from build123d import *

# Parameters (mm, degrees)
F0_W      = 660.4
F0_H      = 304.8
F1_DEPTH  = 6.35
F2_W      = 50.8
F2_H      = 50.8
F3_DEPTH  = 6.35
F4_W      = 50.8
F4_H      = 6.35
F5_W      = 50.8
F5_H      = 6.35
F6_W      = 50.8
F6_H      = 6.35
F7_DEPTH  = 44.45
F8_W      = 101.6
F8_H      = 50.8
F9_DEPTH  = 9.525
F10_W     = 101.6
F10_H     = 50.8
F11_DEPTH = 25.4
F12_W     = 9.525
F12_H     = 50.8
F13_DEPTH = 76.2
F14_W     = 9.525
F14_H     = 50.8
F15_DEPTH = 117.475
F16_R     = 6.35
F17_DEPTH = 25.4
F18_W     = 76.2
F18_H     = 9.525
F19_DEPTH = 76.2
F21_DEPTH = 25.4


with BuildPart() as f1:
    # F0 (on Front) → F1 (new body)
    with BuildSketch(Plane.XZ):
        Rectangle(F0_W, F0_H)
    extrude(amount=F1_DEPTH)

    # F2 (on face) → F3 (join)
    with BuildSketch(Plane.XZ.offset(6.35)):
        with Locations((165.1, -127)):
            Rectangle(F2_W, F2_H)
        with Locations((0, -127)):
            Rectangle(F2_W, F2_H)
        with Locations((-177.8, -127)):
            Rectangle(F2_W, F2_H)
    extrude(amount=F3_DEPTH)

    # F4 (on face) + F5 (on face) + F6 (on face) → F7 (join)
    with BuildSketch(Plane.XZ.offset(12.7)):
        with Locations((-177.8, -149.225)):
            Rectangle(F4_W, F4_H)
    with BuildSketch(Plane.XZ.offset(12.7)):
        with Locations((0, -149.225)):
            Rectangle(F5_W, F5_H)
    with BuildSketch(Plane.XZ.offset(12.7)):
        with Locations((165.1, -149.225)):
            Rectangle(F6_W, F6_H)
    extrude(amount=F7_DEPTH)

    # F8 (on face) → F9 (join)
    with BuildSketch(Plane(origin=(0, 0, 0), x_dir=(-1, 0, 0), z_dir=(0, 1, 0))):
        with Locations((-381, 101.6)):
            Rectangle(F8_W, F8_H)
        with Locations((-279.4, 101.6)):
            Rectangle(F8_W, F8_H)
    extrude(amount=F9_DEPTH)

    # F10 (on face) → F11 (cut)
    with BuildSketch(Plane.XZ.offset(6.35)):
        with Locations((279.4, -127)):
            Rectangle(F10_W, F10_H)
    extrude(amount=-F11_DEPTH, mode=Mode.SUBTRACT)

    # F12 (on face) → F13 (join)
    with BuildSketch(Plane.XZ.offset(6.35)):
        with Locations((300.0375, 101.6)):
            Rectangle(F12_W, F12_H)
    extrude(amount=F13_DEPTH)

    # F14 (on face) → F15 (join)
    with BuildSketch(Plane.YZ.offset(304.8)):
        with Locations((-77.7875, 101.6)):
            Rectangle(F14_W, F14_H)
    extrude(amount=F15_DEPTH)

    # F16 (on face) → F17 (cut)
    with BuildSketch(Plane.XZ.offset(82.55)):
        with Locations((409.575, 101.6)):
            Circle(F16_R)
    extrude(amount=-F17_DEPTH, mode=Mode.SUBTRACT)

    # F18 (on face) → F19 (join)
    with BuildSketch(Plane(origin=(295.275, 0, 0), x_dir=(0, -1, 0), z_dir=(-1, 0, 0))):
        with Locations((44.45, 101.6)):
            Rectangle(F18_W, F18_H)
    extrude(amount=F19_DEPTH)

    # F20 (on face) → F21 (cut)
    with BuildSketch(Plane(origin=(0, 0, 96.8375), x_dir=(1, 0, 0), z_dir=(0, 0, -1))):
        Polygon((219.075, 82.55), (219.075, 6.35), (295.275, 82.55), align=None)
    extrude(amount=-F21_DEPTH, mode=Mode.SUBTRACT)


solid = f1.part
Source: CAD feature listing. Evaluate the final solid. Frame: model axes, mm. A direction names the side the tool comes from. Round coordinates to 2 decimals unless told otherwise and drop trailing zeros. Loops run counter-clockwise (first coordinate to the right, second up) from the corner with the lowest first, then second, coordinate; pieces in that order, holes last. Notation, with made-up numbers: (36.25, 45) - (88.25, 45) arc R7 ccw to (88.25, 55) - close; hole circle Ø7 at (6.25, 45.5). An arc over 180 degrees is marked (long way). Write item = value, one per line. Start each with the question number.
Item 1: Section query A-A on y = -33.5. Count the separate pieces of the cut face and the enclosed holes in it, plus the area to 3 significant figures.
Item 2: First-contact query: pin 1 Ø8 at (x, z) = (-20, 68) entering from -Y; pin 2 Ø13.5 at (x, y) = (-167, -27.5) entering from +Z; pin 3 Ø12 at (y, z) = (-56.5, 101.5) entering from -X (3 decimals). Flat tips, straight axial feed; report the tip coordinate or a pass-through.
Item 3: Reachability of faces 5 (the face through (340, -76, 76.2)), 6 (the face through (266, -35, 96.837)), 7 (the face through (25.4, -20, -148)), 8 (the face through (0, -35, -146.05)) from +Z, -Z, +X, -X, +Y, -Y: full face, straight path, thin tool, end or side. Return the list, or none.
Item 4: Section query D-D on z = -118. Output: boundary loops of the cut face in (x, y), plus the area to 3 significant figures.
Item 5: Section query C-C on x = -274. Output: boundary loops of the cut face in (y, z).
Item 6: Material intervals for line 1 (Y direction, x = -64.5, z = -50); line 2 (Y direction, x = -17, z = -106); line 3 (Z direction, x = 0, y = -39), sorted ascending.
Item 7: Mould query, pull axis Y, two halves, no side actions, for faces 1 (the face through (358, -82.55, 101)), 2 (the face through (-178, -35, -146.05)), 3 (the face through (332, 9.525, 102)), 4 (the face through (304.8, -39, 101)). Classes: released by +Y, released by -Y, zero draft, split by the parting line, or undercut.
Item 8: Section query B-B on z = 87. Output: boundary loops of the cut face in (x, y) (3 decimals), plus the area to 3 significant figures.
Results list:
q1.separate_pieces = 4
q1.enclosed_holes = 0
q1.area = 1,920 mm²
q2.pin_1 = -6.35
q2.pin_2 = -146.05
q2.pin_3 = 263.225
q3.face_5 = -Z, +X, -X, -Y
q3.face_6 = -Z, -X, -Y
q3.face_7 = +Z, -Z, -Y
q3.face_8 = +Z, +X, -X, -Y
q4.outline = (-330.2, -6.35) - (-203.2, -6.35) - (-203.2, -12.7) - (-152.4, -12.7) - (-152.4, -6.35) - (-25.4, -6.35) - (-25.4, -12.7) - (25.4, -12.7) - (25.4, -6.35) - (139.7, -6.35) - (139.7, -12.7) - (190.5, -12.7) - (190.5, -6.35) - (228.6, -6.35) - (228.6, 0) - (-330.2, 0) - close
q4.area = 4,520 mm²
q5.outline = (-6.35, -152.4) - (0, -152.4) - (0, 152.4) - (-6.35, 152.4) - close
q6.line_1 = -6.35 to 0
q6.line_2 = -12.7 to 0
q6.line_3 = -152.4 to -146.05
q7.face_1 = released by -Y
q7.face_2 = zero draft
q7.face_3 = released by +Y
q7.face_4 = undercut
q8.outline = (-330.2, -6.35) - (295.275, -6.35) - (295.275, -82.55) - (422.275, -82.55) - (422.275, -73.025) - (304.8, -73.025) - (304.8, -6.35) - (330.2, -6.35) - (330.2, 0) - (431.8, 0) - (431.8, 9.525) - (228.6, 9.525) - (228.6, 0) - (-330.2, 0) - close
q8.area = 7,970 mm²
